from build123d import *

# Parameters (mm, degrees)
ESBO_O1_W                = 32
ESBO_O1_H                = 35
RESSALTO_EXTRUS_O1_DEPTH = 6
ESBO_O2_R                = 2
ESBO_O2_W                = 12
ESBO_O2_H                = 20
CORTE_EXTRUS_O1_DEPTH    = 6
FILETE1_R                = 5
ESBO_O5_R                = 1.5
CORTE_EXTRUS_O3_DEPTH    = 6
ESBO_O6_R                = 2.5
CORTE_EXTRUS_O4_DEPTH    = 2.4


with BuildPart() as part:
    # Esboço1 → Ressalto-extrusão1 (new body)
    with BuildSketch(Plane.XY):
        Rectangle(ESBO_O1_W, ESBO_O1_H)
    extrude(amount=RESSALTO_EXTRUS_O1_DEPTH)

    # Esboço2 → Corte-extrusão1 (cut)
    with BuildSketch(Plane.XY.offset(6)):
        with Locations((-6, -12.5)):
            Circle(ESBO_O2_R)
        with Locations((-6, -2.5)):
            Circle(ESBO_O2_R)
        with Locations((10, -7.5)):
            Rectangle(ESBO_O2_W, ESBO_O2_H)
    extrude(amount=-CORTE_EXTRUS_O1_DEPTH, mode=Mode.SUBTRACT)

    # Filete1
    filete1_edges = [part.edges().sort_by_distance(p)[0] for p in [
        (4, 2.5, 3),
    ]]
    fillet(filete1_edges, radius=FILETE1_R)

    # Esboço5 → Corte-extrusão3 (cut)
    with BuildSketch(Plane(origin=(0, 0, 0), x_dir=(-1, 0, 0), z_dir=(0, 0, -1))):
        with Locations((-10.8375, 10.9375)):
            Circle(ESBO_O5_R)
        with Locations((-1.3125, 10.9375)):
            Circle(ESBO_O5_R)
    extrude(amount=-CORTE_EXTRUS_O3_DEPTH, mode=Mode.SUBTRACT)

    # Esboço6 → Corte-extrusão4 (cut)
    with BuildSketch(Plane.XY.offset(6)):
        with Locations((10.8375, 10.9375)):
            Circle(ESBO_O6_R)
        with Locations((1.3125, 10.9375)):
            Circle(ESBO_O6_R)
    extrude(amount=-CORTE_EXTRUS_O4_DEPTH, mode=Mode.SUBTRACT)


solid = part.part
The listing builds one solid part. Answer for the finished solid, in the listing's coordinates (mm). A direction names the side the tool comes from. Round coordinates to 2 decimals unless told otherwise and drop trailing zeros. Write each loop counter-clockwise with the first axis right and the second up, starting at its lowest first coordinate (ties: lowest second). Pieces come first, ordered by that corner, then holes. Notation, with made-up numbers: M 2,68.25 L 45,68.25 A27 ccw 45,91.25 Z; hole C 60.5,-32.75 d3. An arc over 180 degrees is marked long. Write each question's results on one line, items separated by ' | '. Start each with the question number.
Item 1: Find section C-C on x = 2. Write down the section's boundary in (y, z).
Item 2: Which of the six approach directions +Z, -Z, +X, -X, +Y, -Y give full straight-line access (tool end or side, diameter ignored) to faces 4 (the cylindrical face through (2.5, 10.02, 1.77)), 5 (the flat face through (12, 2.5, 3)), 6 (the flat face through (1, 9, 3.6))?
Item 3: Given pin 1 Ø4.5 at (x, y) = (-6, -2.5) entering from +Z; pin 2 Ø1.5 at (x, y) = (10, 11) entering from +Z; pin 3 Ø1.8 at (x, z) = (11.5, 4) entering from -Y; pin 4 Ø2 at (x, z) = (5.5, 2) entering from -Y, each flat-ended and moving along its own axis, determine where each tip first touches the part or whether it passes through.
Item 4: Find section A-A on x = -6. Write down the section's boundary in (y, z).
Item 5: Find section D-D on z = 1.75. Write down the section's boundary in (x, y), and give its area (3 significant figures).
Item 6: Straight lines are drawn through the part: probe 1 along Y at (x, z) = (-6, 3); probe 2 along X at (y, z) = (12, 2.8); probe 3 along Y at (x, z) = (11, 2.55). For each, find the intervals that lie inside material, in ascending order.
Item 7: Find section B-B on y = -12.5. Write down the section's boundary in (x, z), and give its area (3 significant figures).
Item 8: The mould has two halves that part along X. Classify faces 1 (the flat face through (4, -10, 3)), 2 (the cylindrical face through (0.771, 8.497, 4.817)), 3 (the flat face through (-16, 0, 3)): +X half, -X half, draft (parallel to the pull), parting line (faces both ways), or undercut.
Answer block:
1) outline: M -17.5,0 L 9.6,0 L 9.6,3.6 L 8.53,3.6 L 8.53,6 L -17.5,6 Z; M 12.27,0 L 17.5,0 L 17.5,6 L 13.34,6 L 13.34,3.6 L 12.27,3.6 Z
2) face 4: +Z, -Z | face 5: +Z, -Z, +X, -Y | face 6: +Z
3) pin 1: stops at z = 6 | pin 2: stops at z = 3.6 | pin 3: stops at y = 2.5 | pin 4: stops at y = -0.32
4) outline: M -17.5,0 L -14.5,0 L -14.5,6 L -17.5,6 Z; M -10.5,0 L -4.5,0 L -4.5,6 L -10.5,6 Z; M -0.5,0 L 17.5,0 L 17.5,6 L -0.5,6 Z
5) outline: M -16,-17.5 L 4,-17.5 L 4,-2.5 A5 cw 9,2.5 L 16,2.5 L 16,17.5 L -16,17.5 Z; hole C -6,-12.5 d4; hole C -6,-2.5 d4; hole C 1.31,10.94 d3; hole C 10.84,10.94 d3 | area: 846 mm²
6) probe 1: y = -17.5 to -14.5, -10.5 to -4.5, -0.5 to 17.5 | probe 2: x = -16 to 0.25, 2.37 to 9.78, 11.9 to 16 | probe 3: y = 2.5 to 9.45, 12.43 to 17.5
7) outline: M -16,0 L -8,0 L -8,6 L -16,6 Z; M -4,0 L 4,0 L 4,6 L -4,6 Z | area: 96.0 mm²
8) face 1: +X half | face 2: undercut | face 3: -X half
